```python
from build123d import *

# Parameters (mm, degrees)
SKETCH1_R                 = 1.6002
SKETCH1_R_2               = 11.5
BOSS_EXTRUDE1_DEPTH       = 6.35
F_6_32_TAPPED_HOLE1_D     = 3.25
F_6_32_TAPPED_HOLE1_DEPTH = 10
F_6_32_TAPPED_HOLE1_TIP   = 0.976398506
REDONDEO1_R               = 15
SKETCH1_4_W               = 10
SKETCH1_4_H               = 10
SALIENTE_EXTRUIR1_DEPTH   = 6.35
CORTAR_EXTRUIR1_REACH     = 118.367
REDONDEO2_R               = 5


with BuildPart() as part:
    # Sketch1 → Boss-Extrude1 (new body)
    with BuildSketch(Plane.XY):
        with BuildLine():
            Line((17.5, -40), (62.5, -40))
            ThreePointArc((62.5, -40), (60.548464977, -33.716680328), (55.380636605, -29.644562334))
            ThreePointArc((55.380636605, -29.644562334), (40.586668907, -17.987290127), (35, 0))
            Line((35, 0), (0, 0))
            Line((0, 0), (0, -40))
            Line((0, -40), (0, -90.8))
            Line((0, -90.8), (9.525, -90.8))
            Line((9.525, -90.8), (62.5, -90.8))
            Line((62.5, -90.8), (62.5, -80.8))
            Line((62.5, -80.8), (9.894504833, -80.8))
            ThreePointArc((9.894504833, -80.8), (12.482988146, -62.642036842), (17.5, -45))
            Line((17.5, -45), (17.5, -40))
        make_face()
        with Locations((4.5, -4.5)):
            Circle(SKETCH1_R, mode=Mode.SUBTRACT)
        with Locations((17.5, -17.5)):
            Circle(SKETCH1_R_2, mode=Mode.SUBTRACT)
        with Locations((30.5, -30.5)):
            Circle(SKETCH1_R, mode=Mode.SUBTRACT)
    extrude(amount=BOSS_EXTRUDE1_DEPTH)

    # #6-32 Tapped Hole1
    with Locations(Plane(origin=(0, -40, 0), x_dir=(-1, 0, 0), z_dir=(0, -1, 0))):
        with Locations((-22.58, -3.175), (-47.98, -3.175)):
            Hole(F_6_32_TAPPED_HOLE1_D / 2, depth=F_6_32_TAPPED_HOLE1_DEPTH)
            with Locations((0, 0, -(F_6_32_TAPPED_HOLE1_DEPTH + F_6_32_TAPPED_HOLE1_TIP / 2))):  # 118° drill point
                Cone(0, F_6_32_TAPPED_HOLE1_D / 2, F_6_32_TAPPED_HOLE1_TIP, mode=Mode.SUBTRACT)

    # Redondeo1
    redondeo1_edges = [part.edges().sort_by_distance(p)[0] for p in [
        (9.894504833, -80.8, 3.175),
    ]]
    fillet(redondeo1_edges, radius=REDONDEO1_R)

    # Sketch1<4> → Saliente-Extruir1 (add)
    with BuildSketch(Plane.XY):
        with Locations((67.5, -85.8)):
            Rectangle(SKETCH1_4_W, SKETCH1_4_H)
    extrude(amount=SALIENTE_EXTRUIR1_DEPTH)

    # Croquis1 → Cortar-Extruir1 (cut, up to next)
    with BuildSketch(Plane.XZ.offset(90.8), mode=Mode.PRIVATE) as cortar_extruir1_sk1:
        with BuildLine():
            ThreePointArc((62.875, 3.175), (64.5, 1.55), (66.125, 3.175))
            Line((66.125, 3.175), (62.875, 3.175))
        make_face()
    cortar_extruir1_tool1 = extrude(cortar_extruir1_sk1.sketch, amount=-CORTAR_EXTRUIR1_REACH, mode=Mode.PRIVATE) & part.part
    # Croquis1 → Cortar-Extruir1 (cut, up to next)
    with BuildSketch(Plane.XZ.offset(90.8), mode=Mode.PRIVATE) as cortar_extruir1_sk2:
        with BuildLine():
            Line((62.875, 3.175), (66.125, 3.175))
            ThreePointArc((66.125, 3.175), (64.5, 4.8), (62.875, 3.175))
        make_face()
    cortar_extruir1_tool2 = extrude(cortar_extruir1_sk2.sketch, amount=-CORTAR_EXTRUIR1_REACH, mode=Mode.PRIVATE) & part.part
    # Croquis1 → Cortar-Extruir1 (cut, up to next)
    with BuildSketch(Plane.XZ.offset(90.8), mode=Mode.PRIVATE) as cortar_extruir1_sk3:
        with BuildLine():
            ThreePointArc((62.875, 3.175), (64.5, 1.55), (66.125, 3.175))
            Line((66.125, 3.175), (62.875, 3.175))
        make_face()
    cortar_extruir1_tool3 = extrude(cortar_extruir1_sk3.sketch, amount=-CORTAR_EXTRUIR1_REACH, mode=Mode.PRIVATE) & part.part
    # Croquis1 → Cortar-Extruir1 (cut, up to next)
    with BuildSketch(Plane.XZ.offset(90.8), mode=Mode.PRIVATE) as cortar_extruir1_sk4:
        with BuildLine():
            Line((62.875, 3.175), (66.125, 3.175))
            ThreePointArc((66.125, 3.175), (64.5, 4.8), (62.875, 3.175))
        make_face()
    cortar_extruir1_tool4 = extrude(cortar_extruir1_sk4.sketch, amount=-CORTAR_EXTRUIR1_REACH, mode=Mode.PRIVATE) & part.part
    add(cortar_extruir1_tool1.solids().sort_by_distance((64.5, -90.8, 2.485329))[0], mode=Mode.SUBTRACT)
    add(cortar_extruir1_tool2.solids().sort_by_distance((64.5, -90.8, 3.864671))[0], mode=Mode.SUBTRACT)
    add(cortar_extruir1_tool3.solids().sort_by_distance((64.5, -90.8, 2.485329))[0], mode=Mode.SUBTRACT)
    add(cortar_extruir1_tool4.solids().sort_by_distance((64.5, -90.8, 3.864671))[0], mode=Mode.SUBTRACT)

    # Redondeo2
    redondeo2_edges = [part.edges().sort_by_distance(p)[0] for p in [
        (0, 0, 3.175),
        (35, 0, 3.175),
    ]]
    fillet(redondeo2_edges, radius=REDONDEO2_R)


solid = part.part
```
The model under review builds one solid part; all positions refer to its coordinate system, in mm. A direction names the side the tool comes from. Give positions to 0.01 mm unless a question says otherwise; leave off trailing zeros. Write each loop counter-clockwise with the first axis right and the second up, starting at its lowest first coordinate (ties: lowest second). Pieces come first, ordered by that corner, then holes.
(1) For P1, Ø10, axis at x = 11.5, y = -44, coming from the -Z side; P2, Ø1.5, axis at y = -42.5, z = 2.5, coming from the +X side, all flat-tipped, find the tip position at first contact; note any pin that passes through.
(2) Consider section B-B, the plane y = -17.5. Give the boundary of the cut face in (x, z), and give its area (3 significant figures).
(3) The part is to be moulded in two halves that separate along Y. For faces 1 (the cylindrical face through (20.957, -34.93, 3.104)), 2 (the cylindrical face through (42.02, -19.91, 3.13)), 3 (the flat face through (36, -90.8, 3)), 4 (the cylindrical face through (62.95, -85.87, 2.69)), say which applies: released by +Y, released by -Y, zero draft, split by the parting line, or undercut.
(4) Consider section A-A, the plane x = 64.5. Give the boundary of the cut face in (y, z), and give its area (3 significant figures).
(5) Tool access review of faces 5 (the flat face through (17.5, -43, 3)), 6 (the cylindrical face through (33.666, -1.265, 3.219)), 7 (the conical face through (47.72, -29.19, 3.28)): name each direction out of +Z, -Z, +X, -X, +Y, -Y from which nothing blocks a thin tool from reaching the whole face with its end or side.
(6) To check wall thickness, follow L1, parallel to Y at x = 24.5, z = 0.5; L2, parallel to Y at x = 30.5, z = 4; L3, parallel to Z at x = 47.98, y = -32. State the ranges of each line that lie inside material, in increasing order.
(7) Consider section C-C, the plane x = 14.5. Give the boundary of the cut face in (y, z), and give its area (3 significant figures).
(8) Consider section D-D, the plane y = -43.5. Give the boundary of the cut face in (x, z), and give its area (3 significant figures).
Returned:
1. P1: stops at z = 0
1. P2: stops at x = 17.5
2. outline: (0, 0) - (6, 0) - (6, 6.35) - (0, 6.35) - close; (29, 0) - (40.26, 0) - (40.26, 6.35) - (29, 6.35) - close
2. area: 110 mm2
3. face 1: undercut
3. face 2: released by +Y
3. face 3: released by -Y
3. face 4: zero draft
4. outline: (-90.8, 0) - (-80.8, 0) - (-80.8, 1.55) - (-90.8, 1.55) - close; (-90.8, 4.8) - (-80.8, 4.8) - (-80.8, 6.35) - (-90.8, 6.35) - close
4. area: 31.0 mm2
5. face 5: +Z, -Z, +X
5. face 6: +Z, -Z, +X, +Y
5. face 7: none
6. L1: y = -90.8 to -80.56, -40 to -26.62, -8.38 to 0
6. L2: y = -90.8 to -80.8, -40 to -32.1, -28.9 to 0
6. L3: z = 0 to 1.55, 4.8 to 6.35
7. outline: (-90.8, 0) - (-73.87, 0) - (-73.87, 6.35) - (-90.8, 6.35) - close; (-54.42, 0) - (-28.6, 0) - (-28.6, 6.35) - (-54.42, 6.35) - close; (-6.4, 0) - (0, 0) - (0, 6.35) - (-6.4, 6.35) - close
7. area: 312 mm2
8. outline: (0, 0) - (17.5, 0) - (17.5, 6.35) - (0, 6.35) - close
8. area: 111 mm2
